Can you work these out from the model? Positions are in its coordinate system, mm. Face numbers are marked on the shaded views. Give positions to 0.01 mm unless a question says otherwise; leave off trailing zeros. Order: outer loops, then holes, each group sorted by start corner. A loop starts at its lowest first (then second) coordinate and runs counter-clockwise, first axis right, second up.
Item 1: If we mould it in two halves opening along Y, with no side actions, what happens to the marked faces 1, 2 and 3? For each: +Y half, -Y half, draft (parallel to the pull), parting line (faces both ways), or undercut.
Item 2: I want a section at C-C, the plane y = 5. Count the separate pieces of the cut face and the enclosed holes in it, then the cut area to 3 significant figures.
Item 3: I want a section at A-A, the plane y = 12.5. Write out the boundary of the cut face in (x, z).
Item 4: I want a section at B-B, the plane x = 5. Write out the boundary of the cut face in (y, z).
Item 5: If I drill on line 1 along Y through (x, z) = (9.75, -25); line 2 along X through (y, z) = (-2.5, -12.5); line 3 along X through (y, z) = (-1.5, -12), over which ranges is the centre line in solid material (lowest first)?
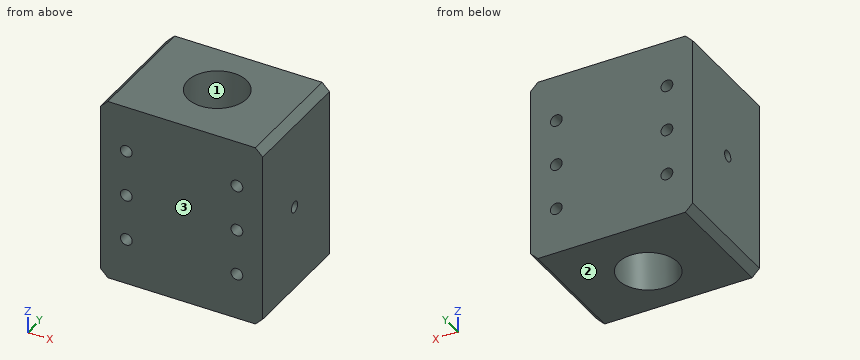
```python
from build123d import *

# Parameters (mm, degrees)
IZIM1_W                     = 44
IZIM1_H                     = 32
Y_KSEKLIK_EKSTR_ZYON1_DEPTH = 50
KES_EKSTR_ZYON1_DEPTH       = 56
KES_EKSTR_ZYON1_DEPTH_BACK  = 60
IZIM2_R                     = 8
IZIM4_R                     = 1.6
KES_EKSTR_ZYON2_DEPTH       = 60
IZIM5_R                     = 1.5
KES_EKSTR_ZYON3_DEPTH       = 45
PAH1_SIZE                   = 2


with BuildPart() as part:
    # Çizim1 → Yükseklik-Ekstrüzyon1 (new body)
    with BuildSketch(Plane.XY):
        Rectangle(IZIM1_W, IZIM1_H)
    extrude(amount=-Y_KSEKLIK_EKSTR_ZYON1_DEPTH)

    # Çizim2 → Kes-Ekstrüzyon1 (cut, two sides: drawn at the far end of the back side and taken through both)
    with BuildSketch(Plane(origin=(0, 0.043824837, 0.836227706), x_dir=(-1, 0, 0), z_dir=(0, 0.05233595624294396, 0.998629534754574)).offset(-KES_EKSTR_ZYON1_DEPTH_BACK)):
        with Locations(Location((0, -1.08, 0), (0, 0, 90))):
            Circle(IZIM2_R)
    extrude(amount=KES_EKSTR_ZYON1_DEPTH + KES_EKSTR_ZYON1_DEPTH_BACK, mode=Mode.SUBTRACT)

    # Çizim4 → Kes-Ekstrüzyon2 (cut)
    with BuildSketch(Plane(origin=(0, 16, 0), x_dir=(1, 0, 0), z_dir=(0, 1, 0))):
        with Locations(Location((-15, 25, 0), (0, 0, 270))):
            Circle(IZIM4_R)
        with Locations(Location((-15, 37.5, 0), (0, 0, 270))):
            Circle(IZIM4_R)
        with Locations(Location((-15, 12.5, 0), (0, 0, 270))):
            Circle(IZIM4_R)
        with Locations(Location((15, 12.5, 0), (0, 0, 270))):
            Circle(IZIM4_R)
        with Locations(Location((15, 37.5, 0), (0, 0, 270))):
            Circle(IZIM4_R)
        with Locations(Location((15, 25, 0), (0, 0, 270))):
            Circle(IZIM4_R)
    extrude(amount=-KES_EKSTR_ZYON2_DEPTH, mode=Mode.SUBTRACT)

    # Çizim5 → Kes-Ekstrüzyon3 (cut, symmetric)
    with BuildSketch(Plane(origin=(0, 0, 0), x_dir=(0, 0, -1), z_dir=(1, 0, 0))):
        with Locations((25, -0.769453415)):
            Circle(IZIM5_R)
    extrude(amount=KES_EKSTR_ZYON3_DEPTH, both=True, mode=Mode.SUBTRACT)

    # Pah1
    pah1_edges = [part.edges().sort_by_distance(p)[0] for p in [
        (-22, 0, -50),
        (22, 0, -50),
        (-22, 0, 0),
        (22, 0, 0),
    ]]
    chamfer(pah1_edges, length=PAH1_SIZE)


solid = part.part
```
Results list:
1. face 1: undercut
1. face 2: draft
1. face 3: -Y half
2. separate pieces: 2
2. enclosed holes: 6
2. area: 1,550 mm2
3. outline: (-22, -48) - (-20, -50) - (20, -50) - (22, -48) - (22, -2) - (20, 0) - (-20, 0) - (-22, -2) - close; hole circle Ø3.2 at (-15, -37.5); hole circle Ø3.2 at (-15, -25); hole circle Ø3.2 at (-15, -12.5); hole circle Ø3.2 at (15, -37.5); hole circle Ø3.2 at (15, -25); hole circle Ø3.2 at (15, -12.5)
4. outline: (-16, -50) - (-7.79, -50) - (-5.17, 0) - (-16, 0) - close; (4.71, -50) - (16, -50) - (16, 0) - (7.34, 0) - close
5. line 1: y = -16 to -2.27, 0.73 to 16
5. line 2: x = -22 to -16.6, -13.4 to -7.45, 7.45 to 13.4, 16.6 to 22
5. line 3: x = -22 to -16.52, -13.48 to -7.76, 7.76 to 13.48, 16.52 to 22
